```python
from build123d import *

# Parameters (mm, degrees)
FILLET1_R = 2


with BuildPart() as part:
    # Sketch1 → Revolve1 (revolve)
    with BuildSketch(Plane.XY):
        with BuildLine():
            Line((15.5, 65), (-15.5, 65))
            Line((-15.5, 65), (-15.5, 53))
            Line((-15.5, 53), (-8.94427191, 53))
            ThreePointArc((-8.94427191, 53), (0, 57), (8.94427191, 53))
            Line((8.94427191, 53), (15.5, 53))
            Line((15.5, 53), (15.5, 65))
        make_face()
    revolve(axis=Axis((-15.5, 0, 0), (1, 0, 0)))

    # Fillet1
    fillet1_edges = [part.edges().sort_by_distance(p)[0] for p in [
        (15.5, -65, 0),
        (-15.5, -65, 0),
    ]]
    fillet(fillet1_edges, radius=FILLET1_R)


solid = part.part
```
Geometry check sheet. Reference: the model listing, model coordinates, mm. Coordinates: 2 decimals unless noted, no trailing zeros. Order: outer loops, then holes, each group sorted by start corner. A loop starts at its lowest first (then second) coordinate and runs counter-clockwise, first axis right, second up. Notation, with made-up numbers: (59.5, 13.5) - (63.5, 13.5) arc R26 cw to (63.5, 28.5) - close; hole circle Ø11 at (13.25, 42.25). An arc over 180 degrees is marked (long way). Answer in a Markdown table with one row per item. Add a question column.
1. Draft check along Z on faces 1 (the face through (12, 28, 45)), 2 (the face through (-15.5, -14, 52)), 3 (the face through (-0.19, 62, 19.52)), 4 (the face through (-12, 28, 45)). Enter one of: +Z half, -Z half, draft (parallel to the pull), parting line (faces both ways), or undercut.
2. Gauge pin test, flat ends, axial feed: pin 1 Ø1.5 at (x, y) = (-0.5, -2) entering from +Z; pin 2 Ø3 at (x, z) = (5.5, 15.5) entering from -Y; pin 3 Ø5 at (x, z) = (1, 35) entering from +Y. Record the tip position at first contact, or that the pin passes through.
3. Section check C-C (x = 0). Enter the section's corners in (y, z), plus the area to 3 significant figures.
4. Material ranges on L1, parallel to Z at x = 13, y = 0; L2, parallel to Y at x = -12.5, z = 1; L3, parallel to Z at x = -10, y = -42, recorded low to high. Write a range as [from, to].
5. Section check A-A (y = 0). Enter the section's corners in (x, z).
Data:
| question | item | result |
|---|---|---|
| 1 | face 1 | undercut |
| 1 | face 2 | draft |
| 1 | face 3 | parting line |
| 1 | face 4 | undercut |
| 2 | pin 1 | stops at z = 64.99 |
| 2 | pin 2 | stops at y = -63.47 |
| 2 | pin 3 | stops at y = 56.29 |
| 3 | outline | circle Ø130 at (0, 0); hole circle Ø114 at (0, 0) |
| 3 | area | 3,070 mm² |
| 4 | L1 | z = [-65, -53], [53, 65] |
| 4 | L2 | y = [-64.99, -52.99], [52.99, 64.99] |
| 4 | L3 | z = [-49.61, -32.33], [32.33, 49.61] |
| 5 | outline | (-15.5, -63) arc R2 ccw to (-13.5, -65) - (13.5, -65) arc R2 ccw to (15.5, -63) - (15.5, -53) - (8.94, -53) arc R12 cw to (-8.94, -53) - (-15.5, -53) - close; (-15.5, 53) - (-8.94, 53) arc R12 cw to (8.94, 53) - (15.5, 53) - (15.5, 63) arc R2 ccw to (13.5, 65) - (-13.5, 65) arc R2 ccw to (-15.5, 63) - close |
